Design review of the part built by this model. Coordinates are the model's own, in mm. A direction names the side the tool comes from. Round coordinates to 2 decimals unless told otherwise and drop trailing zeros. Write each loop counter-clockwise with the first axis right and the second up, starting at its lowest first coordinate (ties: lowest second). Pieces come first, ordered by that corner, then holes. Notation, with made-up numbers: (5, -26.5) - (62, -26.5) arc R31 ccw to (62, 7.5) - close; hole circle Ø2 at (82, 87.5). An arc over 180 degrees is marked (long way). Use one line per item in the form item = value.
Autodesk Inventor part; units mm, degrees
ref_plane "YZ Plane" through (0, 0, 0) normal (1, 0, 0) x (0, 1, 0)
ref_plane "XZ Plane" through (0, 0, 0) normal (0, 1, 0) x (-1, 0, 0)
ref_plane "XY Plane" through (0, 0, 0) normal (0, 0, 1) x (1, 0, 0)
sketch "スケッチ1" plane through (0, 0, 0) normal (0, 1, 0) x (-1, 0, 0)
  circle A0 centre (0, 0) radius 1.15
  circle A1 centre (0, 0) radius 3.1
  circle A2 centre (0, 0) radius 4.9
  line L0 (3.1, 0) -> (8.1, 0)
  line L1 (8.1, 0) -> (8.1, 10)
  line L2 (8.1, 10) -> (3.1, 10)
  line L3 (3.1, 10) -> (3.1, 0)
  line L4 (0, 0) -> (0, 4.9)
  line L5 (0, 4.9) -> (3.1, 5)
  line L6 (8.1, 0) -> (2.9642, -3.9017)
  circle A3 centre (0, 0) radius 2
  line L7 (0, -2) -> (-4.4733, -2)
  line L8 (8.1, 0) -> (8.1, -4.9)
  line L9 (8.1, -4.9) -> (0, -4.9)
  point P0 (-2.3685, -2)
  dimension "d1" = 6.2
  dimension "d5" = 4
  dimension "d0" = 2.3
  dimension "d2" = 9.8
  dimension "d3" = 5
  dimension "d4" = 10
extrude "押し出し1" add sketch "スケッチ1" along normal blind 6.65 contours L0 A2 L7 A1 | L3 A2 L0 | L0 L6 A2 | A2 L3 L2 L1 L0 | L6 L8 L9 A2
extrude "押し出し2" add sketch "スケッチ1" against normal blind 1.1
sketch "スケッチ2" plane through (0, 6.65, 0) normal (0, 1, 0) x (1, 0, 0)
  circle A0 centre (0, 0) radius 1.15
  circle A1 centre (0, 0) radius 1.15
  arc A2 (2.3685, 2) -> (-3.1, 0) centre (0, 0) ccw
  circle A3 centre (0, 0) radius 4.9
  line L0 (-8.1, -10) -> (-8.1, 4.9)
  line L1 (-3.1, 0) -> (-8.1, 0)
  line L2 (-8.1, 0) -> (-8.1, -10)
  line L3 (-8.1, -10) -> (-3.1, -10)
  line L4 (-3.1, -10) -> (-3.1, 0)
  line L5 (-3.1, -5) -> (0, -4.9)
  line L6 (0, -4.9) -> (-3.1, -5)
  line L7 (-3.1, -5) -> (-3.1, 0)
  line L8 (0, 0) -> (-8.1, 0)
  line L9 (-8.1, 0) -> (-8.1, 4.9)
  line L10 (-8.1, 4.9) -> (0, 4.9)
  line L11 (0, 4.9) -> (0, 0)
  dimension "d11" = 9.8
  dimension "d10" = 2.3
  dimension "d12" = 5
  dimension "d13" = 10
extrude "押し出し3" add sketch "スケッチ2" along normal blind 1.1 contours A0 L11 A3 L4 L8 | A0 L8 A2 L11 | A2 L1 A3 L11 | L4 A3 L1 | A3 L1 L0 L10 | A3 L4 L3 L0 L1 | A3 L5 L4
sketch "スケッチ3" plane through (-8.1, -1.1, 10) normal (0, 0, 1) x (1, 0, 0)
  line L0 (0, 0) -> (8.1, 0)
  line L1 (0, 0) -> (2.5, 0)
  line L2 (2.5, 0) -> (2.5, 4.425)
  line L3 (2.5, 4.425) -> (0, 4.425)
  line L4 (0, 4.425) -> (0, 0)
  circle A0 centre (2.5, 4.425) radius 1.6
  point P0 (8.1, 1.1)
  dimension "d16" = 2.5
  dimension "d17" = 4.425
  dimension "d18" = 3.2
extrude "押し出し4" cut sketch "スケッチ3" against normal blind 10 contours A0 L3 L2 | L2 L3 A0
properties part number "srod2.1"
Q1. We need section C-C on x = -5.6. Write out the cut boundary in (y, z) (3 decimals), then the cut area to 3 significant figures.
Calculated:
outline = (-1.1, -4.9) - (7.75, -4.9) - (7.75, 10) - (4.925, 10) - (4.925, 0) - (1.725, 0) - (1.725, 10) - (-1.1, 10) - close
area = 99.9 mm2
Q2. We need section A-A on y = 7. Write out the cut boundary in (x, z).
Calculated:
outline = (-8.1, -4.9) - (0, -4.9) arc R4.9 ccw to (0, 4.9) - (-3.1, 5) - (-3.1, 10) - (-8.1, 10) - close; hole circle Ø2.3 at (0, 0)
Q3. We need section B-B on x = -0.25. Write out the cut boundary in (y, z).
Calculated:
outline = (-1.1, -4.9) - (7.75, -4.9) - (7.75, -1.12) - (6.65, -1.12) - (6.65, -3.09) - (0, -3.09) - (0, -1.12) - (-1.1, -1.12) - close; (-1.1, 1.12) - (0, 1.12) - (0, 4.91) - (-1.1, 4.91) - close; (6.65, 1.12) - (7.75, 1.12) - (7.75, 4.91) - (6.65, 4.91) - close
Q4. We need section D-D on z = 3. Write out the cut boundary in (x, y) (3 decimals).
Calculated:
outline = (-8.1, -1.1) - (3.874, -1.1) - (3.874, 0) - (-3.1, 0) - (-3.1, 6.65) - (3.874, 6.65) - (3.874, 7.75) - (-8.1, 7.75) - close; hole circle Ø3.2 at (-5.6, 3.325)
Q5. To check wall thickness, follow line 1 along Z through (x, y) = (0, -0.9); line 2 along Y through (x, z) = (0.25, 1.25); line 3 along X through (y, z) = (-0.8, 0). State the ranges of each line that lie inside material, in increasing order. Write a range as from..to.
Calculated:
line_1 = -4.9..-1.15, 1.15..4.9
line_2 = -1.1..0, 6.65..7.75
line_3 = -8.1..-1.15, 1.15..4.9
Q6. Machinability: for faces 4 (the cylindrical face through (-0.91, 7.19, -0.7)), 5 (the cylindrical face through (-1.1, 3.3, -2.9)), 6 (the flat face through (-3.1, 3, 5)), which of the approach directions +Z, -Z, +X, -X, +Y, -Y give a long, thin tool a straight path to every point of the face, cutting with its end or side? Answer none if there is none.
Calculated:
face_4 = +Y, -Y
face_5 = +Z
face_6 = +Z, +X
Q7. Draft analysis for pull direction Z (two halves, no side actions). For faces 1 (the cylindrical face through (-6.87, 2.35, 5.07)), 2 (the cylindrical face through (0.91, -0.54, -0.7)), 3 (the flat face through (-6, 3, 0)), state which applies: released by +Z, released by -Z, zero draft, split by the parting line, or undercut.
Calculated:
face_1 = zero draft
face_2 = undercut
face_3 = released by +Z
Q8. For P1, Ø2.5, axis at x = 3.5, y = 4, coming from the +Z side; P2, Ø6.5, axis at x = 1, z = -0.5, coming from the -Y side; P3, Ø1.5, axis at x = 3, y = 0.5, coming from the +Z side; P4, Ø1.5, axis at y = 1, z = 0, coming from the +X side, all flat-tipped, find the tip position at first contact; note any pin that passes through.
Calculated:
P1 = -2
P2 = -1.1
P3 = 4.25
P4 = -3.01
